Geometry: final body of the model. Coordinates: model frame, mm. A direction names the side the tool comes from. Round coordinates to 2 decimals unless told otherwise and drop trailing zeros. Loops run counter-clockwise (first coordinate to the right, second up) from the corner with the lowest first, then second, coordinate; pieces in that order, holes last. Notation, with made-up numbers: (13, -13.75) - (58, -13.75) arc R8 cw to (58, -6.75) - close; hole circle Ø6 at (34.5, 52.25). An arc over 180 degrees is marked (long way). Answer in a Markdown table with one row per item. Add a question column.
from build123d import *

# Parameters (mm, degrees)
SKETCH2_W           = 150
SKETCH2_H           = 150
BOSS_EXTRUDE1_DEPTH = 225
CUT_EXTRUDE1_DEPTH  = 150
CUT_EXTRUDE2_DEPTH  = 150


with BuildPart() as part:
    # Sketch2 → Boss-Extrude1 (new body)
    with BuildSketch(Plane(origin=(0, 0, 0), x_dir=(0, 0, -1), z_dir=(1, 0, 0))):
        Rectangle(SKETCH2_W, SKETCH2_H)
    extrude(amount=BOSS_EXTRUDE1_DEPTH)

    # Sketch3 → Cut-Extrude1 (cut)
    with BuildSketch(Plane(origin=(0, 75, 0), x_dir=(1, 0, 0), z_dir=(0, 1, 0))):
        Polygon((0, 25), (25, 25), (25, 50), (50, 50), (50, 25), (75, 25), (75, 75), (0, 75), align=None)
        Polygon((75, -25), (50, -25), (50, -50), (25, -50), (25, -25), (0, -25), (0, -75), (75, -75), align=None)
    extrude(amount=-CUT_EXTRUDE1_DEPTH, mode=Mode.SUBTRACT)

    # Sketch4 → Cut-Extrude2 (cut)
    with BuildSketch(Plane.XY.offset(75)):
        Polygon((225, 25), (200, 25), (200, 50), (175, 50), (175, 25), (150, 25), (150, 0), (149.856793805, 0), (149.856793805, -0.1270597), (150, -0.1270597), (150, -25), (175, -25), (175, -50), (200, -50), (200, -25), (225, -25), align=None)
    extrude(amount=-CUT_EXTRUDE2_DEPTH, mode=Mode.SUBTRACT)


solid = part.part
1) Section C-C, the plane y = -47. Return the cut outline in (x, z).
2) Section B-B, the plane z = -34. Return the cut outline in (x, y), and give its area (4 significant figures).
3) Material intervals for line 1 along Y through (x, z) = (195, -54); line 2 along X through (y, z) = (-39.5, -49.5); line 3 along X through (y, z) = (-31, 51.5), sorted ascending. Write a range as from..to.
4) Section A-A, the plane x = 193.5. Return the cut outline in (y, z), and give its area (3 significant figures).
5) Pull-direction query (Y, two-part tool) for faces 1 (the flat face through (136, 75, 1)), 2 (the flat face through (132, -1, -75)), 3 (the flat face through (213, 25, 1)); classes: pulls with the +Y half, pulls with the -Y half, needs draft (parallel to the pull), parting line crosses it, or undercut.
6) Reachability of faces 4 (the flat face through (62, 1, -25)), 5 (the flat face through (188, 50, 1)), 6 (the flat face through (37, 1, -50)), 7 (the flat face through (50, 1, 37)) from +Z, -Z, +X, -X, +Y, -Y: full face, straight path, thin tool, end or side. Return the list, or none.
7) Contact query for flat-ended pins moving along their axis: pin 1 Ø20 at (x, y) = (62.5, -19.5) entering from -Z; pin 2 Ø12.5 at (y, z) = (-21, -34) entering from -X; pin 3 Ø12.5 at (x, y) = (41, 5.5) entering from -Z. Output: stop coordinate, or through.
8) Section D-D, the plane z = -4. Return the cut outline in (x, y), and give its area (4 significant figures).
Evaluation:
| question | item | result |
|---|---|---|
| 1 | outline | (0, -25) - (25, -25) - (25, -50) - (50, -50) - (50, -25) - (75, -25) - (75, -75) - (175, -75) - (175, 75) - (75, 75) - (75, 25) - (50, 25) - (50, 50) - (25, 50) - (25, 25) - (0, 25) - close; (200, -75) - (225, -75) - (225, 75) - (200, 75) - close |
| 2 | outline | (25, -75) - (50, -75) - (50, 75) - (25, 75) - close; (75, -75) - (225, -75) - (225, -25) - (200, -25) - (200, -50) - (175, -50) - (175, -25) - (150, -25) - (150, -0.13) - (149.86, -0.13) - (149.86, 0) - (150, 0) - (150, 25) - (175, 25) - (175, 50) - (200, 50) - (200, 25) - (225, 25) - (225, 75) - (75, 75) - close |
| 2 | area | 21,250 mm² |
| 3 | line 1 | y = -75..-50, 50..75 |
| 3 | line 2 | x = 25..50, 75..175, 200..225 |
| 3 | line 3 | x = 75..175, 200..225 |
| 4 | outline | (-75, -75) - (-50, -75) - (-50, 75) - (-75, 75) - close; (50, -75) - (75, -75) - (75, 75) - (50, 75) - close |
| 4 | area | 7,500 mm² |
| 5 | face 1 | pulls with the +Y half |
| 5 | face 2 | needs draft |
| 5 | face 3 | undercut |
| 6 | face 4 | -Z, +Y, -Y |
| 6 | face 5 | +Z, -Z |
| 6 | face 6 | -Z, -X, +Y, -Y |
| 6 | face 7 | +Z, +Y, -Y |
| 7 | pin 1 | stops at z = -25 |
| 7 | pin 2 | stops at x = 25 |
| 7 | pin 3 | stops at z = -50 |
| 8 | outline | (0, -75) - (225, -75) - (225, -25) - (200, -25) - (200, -50) - (175, -50) - (175, -25) - (150, -25) - (150, -0.13) - (149.86, -0.13) - (149.86, 0) - (150, 0) - (150, 25) - (175, 25) - (175, 50) - (200, 50) - (200, 25) - (225, 25) - (225, 75) - (0, 75) - close |
| 8 | area | 28,750 mm² |
